from build123d import *

# Parameters (mm, degrees)
BOSS_EXTRUDE1_DEPTH       = 100
SKETCH2_W                 = 60
SKETCH2_H                 = 60
BOSS_EXTRUDE2_DEPTH       = 70
CUT_EXTRUDE2_DEPTH        = 60
CUT_EXTRUDE3_DEPTH        = 60
M6_CLEARANCE_HOLE1_REACH  = 177.214
M6_CLEARANCE_HOLE1_BORE_R = 3.3
FILLET1_R                 = 20
FILLET2_R                 = 5


with BuildPart() as part:
    # Sketch1 → Boss-Extrude1 (new body)
    with BuildSketch(Plane.XY):
        with BuildLine():
            Line((25.019, 21.05025), (25.019, -21.05025))
            ThreePointArc((25.019, -21.05025), (23.856580038, -23.856580038), (21.05025, -25.019))
            Line((21.05025, -25.019), (-21.05025, -25.019))
            ThreePointArc((-21.05025, -25.019), (-23.856580038, -23.856580038), (-25.019, -21.05025))
            Line((-25.019, -21.05025), (-25.019, 21.05025))
            ThreePointArc((-25.019, 21.05025), (-23.856580038, 23.856580038), (-21.05025, 25.019))
            Line((-21.05025, 25.019), (21.05025, 25.019))
            ThreePointArc((21.05025, 25.019), (23.856580038, 23.856580038), (25.019, 21.05025))
        make_face()
    extrude(amount=BOSS_EXTRUDE1_DEPTH)

    # Sketch2 → Boss-Extrude2 (add)
    with BuildSketch(Plane.XY):
        Rectangle(SKETCH2_W, SKETCH2_H)
    extrude(amount=-BOSS_EXTRUDE2_DEPTH)

    # Sketch3 → Cut-Extrude2 (cut)
    with BuildSketch(Plane.XZ.offset(30)):
        with BuildLine():
            ThreePointArc((17.5, -25), (-10.458250332, -10.9687848), (-5, -41.770509831))
            Line((-5, -41.770509831), (-5, -38.5))
            Line((-5, -38.5), (5, -38.5))
            Line((5, -38.5), (5, -41.770509831))
            ThreePointArc((5, -41.770509831), (14.0312152, -35.458250332), (17.5, -25))
        make_face()
        with BuildLine():
            Line((-5, -38.5), (-5, -41.770509831))
            ThreePointArc((-5, -41.770509831), (0, -42.5), (5, -41.770509831))
            Line((5, -41.770509831), (5, -38.5))
            Line((5, -38.5), (-5, -38.5))
        make_face()
    extrude(amount=-CUT_EXTRUDE2_DEPTH, mode=Mode.SUBTRACT)

    # Sketch3<7> → Cut-Extrude3 (cut)
    with BuildSketch(Plane.XZ.offset(30)):
        with BuildLine():
            Line((-5, -41.770509831), (-5, -46.5))
            Line((-5, -46.5), (5, -46.5))
            Line((5, -46.5), (5, -41.770509831))
            ThreePointArc((5, -41.770509831), (0, -42.5), (-5, -41.770509831))
        make_face()
    extrude(amount=-CUT_EXTRUDE3_DEPTH, mode=Mode.SUBTRACT)

    # M6 Clearance Hole1 bore → M6 Clearance Hole1 (cut, up to next)
    with BuildSketch(Plane(origin=(0, 0, -70), x_dir=(-1, 0, 0), z_dir=(0, 0, -1)), mode=Mode.PRIVATE) as m6_clearance_hole1_sk1:
        with Locations((0, 20)):
            Circle(M6_CLEARANCE_HOLE1_BORE_R)
    m6_clearance_hole1_tool1 = extrude(m6_clearance_hole1_sk1.sketch, amount=-M6_CLEARANCE_HOLE1_REACH, mode=Mode.PRIVATE) & part.part
    # M6 Clearance Hole1 bore → M6 Clearance Hole1 (cut, up to next)
    with BuildSketch(Plane(origin=(0, 0, -70), x_dir=(-1, 0, 0), z_dir=(0, 0, -1)), mode=Mode.PRIVATE) as m6_clearance_hole1_sk2:
        Circle(M6_CLEARANCE_HOLE1_BORE_R)
    m6_clearance_hole1_tool2 = extrude(m6_clearance_hole1_sk2.sketch, amount=-M6_CLEARANCE_HOLE1_REACH, mode=Mode.PRIVATE) & part.part
    # M6 Clearance Hole1 bore → M6 Clearance Hole1 (cut, up to next)
    with BuildSketch(Plane(origin=(0, 0, -70), x_dir=(-1, 0, 0), z_dir=(0, 0, -1)), mode=Mode.PRIVATE) as m6_clearance_hole1_sk3:
        with Locations((0, -20)):
            Circle(M6_CLEARANCE_HOLE1_BORE_R)
    m6_clearance_hole1_tool3 = extrude(m6_clearance_hole1_sk3.sketch, amount=-M6_CLEARANCE_HOLE1_REACH, mode=Mode.PRIVATE) & part.part
    add(m6_clearance_hole1_tool1.solids().sort_by_distance((0, 20, -70))[0], mode=Mode.SUBTRACT)
    add(m6_clearance_hole1_tool2.solids().sort_by_distance((0, 0, -70))[0], mode=Mode.SUBTRACT)
    add(m6_clearance_hole1_tool3.solids().sort_by_distance((0, -20, -70))[0], mode=Mode.SUBTRACT)

    # Fillet1
    fillet1_edges = [part.edges().sort_by_distance(p)[0] for p in [
        (-30, 0, -70),
        (30, 0, -70),
    ]]
    fillet(fillet1_edges, radius=FILLET1_R)

    # Fillet2
    fillet2_edges = [part.edges().sort_by_distance(p)[0] for p in [
        (-30, 0, 0),
        (0, -30, 0),
        (30, 0, 0),
        (0, 30, 0),
    ]]
    fillet(fillet2_edges, radius=FILLET2_R)


solid = part.part
CAD build for the part. Positions are in the model's coordinates, mm. A direction names the side the tool comes from. Give positions to 0.01 mm unless a question says otherwise; leave off trailing zeros. Loops run counter-clockwise (first coordinate to the right, second up) from the corner with the lowest first, then second, coordinate; pieces in that order, holes last. Notation, with made-up numbers: M 16,76 L 27,76 A23 cw 27,103 Z; hole C -21.75,-33.75 d4. An arc over 180 degrees is marked long. Answer in a Markdown table with one row per item. Add a question column.
Item 1: Probe probe 1 along Y at (x, z) = (0, -61); probe 2 along Z at (x, y) = (0, -15); probe 3 along X at (y, z) = (18.5, -26). List the from-to ranges inside material, lowest first.
Item 2: Band-saw the part on C-C on z = -37.5. Give the cut face in (x, y), then the cut area to 3 significant figures.
Item 3: Drop flat-ended pins along their axis: P1, Ø2, axis at y = -1.5, z = 35.5, coming from the +X side; P2, Ø10, axis at y = 21.5, z = 54.5, coming from the -X side; P3, Ø12.5, axis at x = 5, z = 37.5, coming from the +Y side; P4, Ø21, axis at x = 0, z = -25, coming from the -Y side. Give the stop position or say it passes through.
Item 4: Band-saw the part on A-A on z = 85. Give the cut face in (x, y).
Item 5: Tool access for faces 1 (the face through (23.887, -23.826, 49.3)), 2 (the face through (-24, 24, 0)), 3 (the face through (0, 25.019, 49)), 4 (the face through (-25.019, 0, 49)), 5 (the face through (-23.826, -23.887, 49.3)): list every direction of +Z, -Z, +X, -X, +Y, -Y with a clear straight run to the whole face (end or side of a thin tool).
Item 6: Mould opens along Z. For faces 6 (the face through (0.72, -23.22, -58.41)), 7 (the face through (-29, 25, -2)), 8 (the face through (-5, 0, -44)) say: +Z half, -Z half, draft (parallel to the pull), parting line (faces both ways), or undercut.
Item 7: Band-saw the part on B-B on x = 0. Give the number of separate pieces and of enclosed holes in the cut face, then the cut area to 3 significant figures.
Reply:
| question | item | result |
|---|---|---|
| 1 | probe 1 | y = -30 to -23.3, -16.7 to -3.3, 3.3 to 16.7, 23.3 to 30 |
| 1 | probe 2 | z = -70 to -46.5, -7.5 to 100 |
| 1 | probe 3 | x = -30 to -17.47, 17.47 to 30 |
| 2 | outline | M -30,-30 L -12.25,-30 L -12.25,30 L -30,30 Z; M 12.25,-30 L 30,-30 L 30,30 L 12.25,30 Z |
| 2 | area | 2,130 mm^2 |
| 3 | P1 | stops at x = 25.02 |
| 3 | P2 | stops at x = -25.02 |
| 3 | P3 | stops at y = 25.02 |
| 3 | P4 | passes through |
| 4 | outline | M -25.02,-21.05 A3.97 ccw -21.05,-25.02 L 21.05,-25.02 A3.97 ccw 25.02,-21.05 L 25.02,21.05 A3.97 ccw 21.05,25.02 L -21.05,25.02 A3.97 ccw -25.02,21.05 Z |
| 5 | face 1 | +Z, +X, -Y |
| 5 | face 2 | +Z, -X, +Y |
| 5 | face 3 | +Z, +X, -X, +Y |
| 5 | face 4 | +Z, -X, +Y, -Y |
| 5 | face 5 | +Z, -X, -Y |
| 6 | face 6 | draft |
| 6 | face 7 | +Z half |
| 6 | face 8 | undercut |
| 7 | separate pieces | 5 |
| 7 | enclosed holes | 0 |
| 7 | area | 6,390 mm^2 |
